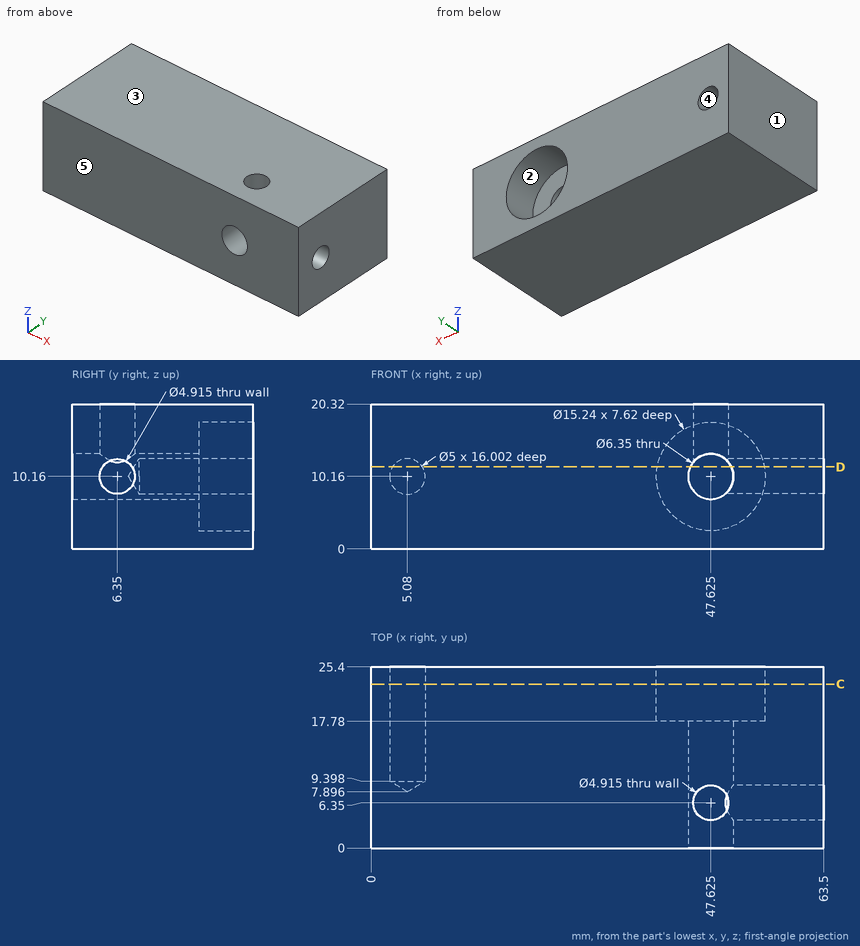
Geometry check sheet. Reference: drawing and pictorial views, mm from the part's lowest x, y, z. A direction names the side the tool comes from. Coordinates: 2 decimals unless noted, no trailing zeros. Write each loop counter-clockwise with the first axis right and the second up, starting at its lowest first coordinate (ties: lowest second). Pieces come first, ordered by that corner, then holes. Notation, with made-up numbers: (-22.75, 52.25) - (11.25, 52.25) arc R34 cw to (11.25, 83.25) - close; hole circle Ø11 at (72, 67.5). An arc over 180 degrees is marked (long way). Write item = value, one per line.
Q1. Material ranges on L1, parallel to X at y = 18.75, z = 10.16 (3 decimals); L2, parallel to X at y = 14.75, z = 10.16; L3, parallel to Z at x = 5.5, y = 12, recorded low to high. Write a range as from..to.
Answer:
L1 = 0..2.58, 7.58..40.005, 55.245..63.5
L2 = 0..2.58, 7.58..44.45, 50.8..63.5
L3 = 0..7.7, 12.62..20.32
Q2. Cross-section at C-C (y = 23). Enter the section's corners in (x, z) (3 decimals).
Answer:
outline = (0, 0) - (63.5, 0) - (63.5, 20.32) - (0, 20.32) - close; hole circle Ø5 at (5.08, 10.16); hole circle Ø15.24 at (47.625, 10.16)
Q3. Mould release check, pull along Z, two halves, no side actions. Record for the marked faces 3, 4 and 5: released by +Z, released by -Z, zero draft, split by the parting line, or undercut.
Answer:
face_3 = released by +Z
face_4 = undercut
face_5 = zero draft
Q4. Go/stop test with flat-tipped pins: pin 1 Ø12 at (x, z) = (47.625, 10.16) entering from +Y; pin 2 Ø4.5 at (x, y) = (47.625, 6.35) entering from +Z. Record where each tip stops, or that it passes through.
Answer:
pin_1 = 17.78
pin_2 = 7.92
Q5. Cross-section at D-D (z = 11.5). Give the number of separate pieces and of enclosed holes in the cut face, plus the area to 3 significant figures.
Answer:
separate_pieces = 3
enclosed_holes = 0
area = 1,270 mm²
Q6. Access from +Z, -Z, +X, -X, +Y, -Y to the whole of each face (thin tool, end or side, straight path). Record for the marked faces 1 and 2.
Answer:
face_1 = +Z, -Z, -X, +Y, -Y
face_2 = +Y
